Geometry check sheet. Reference: the model listing, model coordinates, mm. A direction names the side the tool comes from. Round coordinates to 2 decimals unless told otherwise and drop trailing zeros. Write each loop counter-clockwise with the first axis right and the second up, starting at its lowest first coordinate (ties: lowest second). Pieces come first, ordered by that corner, then holes. Notation, with made-up numbers: M -2,85 L 53,85 A29 cw 53,106 Z; hole C 26.5,-22.5 d8. An arc over 180 degrees is marked long. Use a Markdown table: item, result.
```python
from build123d import *

# Parameters (mm, degrees)
BOSS_EXTRUDE1_DEPTH = 34
SKETCH4_R           = 11
BOSS_EXTRUDE2_DEPTH = 1.5
SKETCH5_W           = 15
SKETCH5_H           = 6
BOSS_EXTRUDE3_DEPTH = 6
SKETCH6_R           = 9
CUT_EXTRUDE1_DEPTH  = 2
SKETCH7_R           = 2.5
BOSS_EXTRUDE4_DEPTH = 20
CUT_EXTRUDE3_DEPTH  = 20
FILLET1_R           = 1
FILLET2_R           = 1
SKETCH9_R           = 1.5
CUT_EXTRUDE4_DEPTH  = 20


with BuildPart() as part:
    # Sketch2 → Boss-Extrude1 (new body)
    with BuildSketch(Plane.XY):
        with BuildLine():
            Line((-16, -21), (16, -21))
            ThreePointArc((16, -21), (19.535533906, -19.535533906), (21, -16))
            Line((21, -16), (21, 16))
            ThreePointArc((21, 16), (19.535533906, 19.535533906), (16, 21))
            Line((16, 21), (-16, 21))
            ThreePointArc((-16, 21), (-19.535533906, 19.535533906), (-21, 16))
            Line((-21, 16), (-21, -16))
            ThreePointArc((-21, -16), (-19.535533906, -19.535533906), (-16, -21))
        make_face()
    extrude(amount=BOSS_EXTRUDE1_DEPTH)

    # Sketch4 → Boss-Extrude2 (add)
    with BuildSketch(Plane.XY.offset(34)):
        Circle(SKETCH4_R)
    extrude(amount=BOSS_EXTRUDE2_DEPTH)

    # Sketch5 → Boss-Extrude3 (add)
    with BuildSketch(Plane.XZ.offset(21)):
        with Locations((0, 7)):
            Rectangle(SKETCH5_W, SKETCH5_H)
    extrude(amount=BOSS_EXTRUDE3_DEPTH)

    # Sketch6 → Cut-Extrude1 (cut)
    with BuildSketch(Plane.XY.offset(35.5)):
        Circle(SKETCH6_R)
    extrude(amount=-CUT_EXTRUDE1_DEPTH, mode=Mode.SUBTRACT)

    # Sketch7 → Boss-Extrude4 (add)
    with BuildSketch(Plane.XY.offset(33.5)):
        Circle(SKETCH7_R)
    extrude(amount=BOSS_EXTRUDE4_DEPTH)

    # Sketch8 → Cut-Extrude3 (cut)
    with BuildSketch(Plane.XY.offset(27)):
        with BuildLine():
            Line((16, 21), (-16, 21))
            ThreePointArc((-16, 21), (-19.535533906, 19.535533906), (-21, 16))
            Line((-21, 16), (-21, -16))
            ThreePointArc((-21, -16), (-19.535533906, -19.535533906), (-16, -21))
            Line((-16, -21), (16, -21))
            ThreePointArc((16, -21), (19.535533906, -19.535533906), (21, -16))
            Line((21, -16), (21, 16))
            ThreePointArc((21, 16), (19.535533906, 19.535533906), (16, 21))
        make_face()
        with BuildLine():
            Line((16, 20.9), (-16, 20.9))
            ThreePointArc((-16, 20.9), (-19.464823228, 19.464823228), (-20.9, 16))
            Line((-20.9, 16), (-20.9, -16))
            ThreePointArc((-20.9, -16), (-19.464823228, -19.464823228), (-16, -20.9))
            Line((-16, -20.9), (16, -20.9))
            ThreePointArc((16, -20.9), (19.464823228, -19.464823228), (20.9, -16))
            Line((20.9, -16), (20.9, 16))
            ThreePointArc((20.9, 16), (19.464823228, 19.464823228), (16, 20.9))
        make_face(mode=Mode.SUBTRACT)
    extrude(amount=-CUT_EXTRUDE3_DEPTH, mode=Mode.SUBTRACT)

    # Fillet1
    fillet1_edges = [part.edges().sort_by_distance(p)[0] for p in [
        (-21, 0, 0),
        (-19.535533906, 19.535533906, 0),
        (0, 21, 0),
        (19.535533906, 19.535533906, 0),
        (-19.535533906, 19.535533906, 34),
        (-21, 0, 34),
        (-19.535533906, -19.535533906, 34),
        (0, -21, 34),
        (19.535533906, -19.535533906, 34),
        (21, 0, 34),
        (19.535533906, 19.535533906, 34),
        (21, 0, 0),
        (0, 21, 34),
        (19.535533906, -19.535533906, 0),
        (0, -21, 0),
        (-19.535533906, -19.535533906, 0),
    ]]
    fillet(fillet1_edges, radius=FILLET1_R)

    # Fillet2
    fillet2_edges = [part.edges().sort_by_distance(p)[0] for p in [
        (-2.5, 0, 53.5),
    ]]
    fillet(fillet2_edges, radius=FILLET2_R)

    # Sketch9 → Cut-Extrude4 (cut)
    with BuildSketch(Plane.XY.offset(34)):
        with Locations((15.5, 15.5)):
            Circle(SKETCH9_R)
        with Locations((15.5, -15.5)):
            Circle(SKETCH9_R)
        with Locations((-15.5, -15.5)):
            Circle(SKETCH9_R)
        with Locations((-15.5, 15.5)):
            Circle(SKETCH9_R)
    extrude(amount=-CUT_EXTRUDE4_DEPTH, mode=Mode.SUBTRACT)


solid = part.part
```
Item 1: Mould release check, pull along Y, two halves, no side actions. Record for faces 4 (the face through (20, 19, 4)), 5 (the face through (21, 0, 4)), 6 (the face through (19, -20, 30)), 7 (the face through (15, -15, 14)): +Y half, -Y half, draft (parallel to the pull), parting line (faces both ways), or undercut.
Outcome:
| item | result |
|---|---|
| face 4 | +Y half |
| face 5 | draft |
| face 6 | -Y half |
| face 7 | undercut |
Item 2: Access from +Z, -Z, +X, -X, +Y, -Y to the whole of each face (thin tool, end or side, straight path). Record for faces 1 (the face through (-19.5, -19.43, 17.14)), 2 (the face through (20.9, 0, 17)), 3 (the face through (7.5, -24, 7)).
Outcome:
| item | result |
|---|---|
| face 1 | -X, -Y |
| face 2 | +X, +Y, -Y |
| face 3 | +Z, -Z, +X, -Y |
Item 3: Material ranges on line 1 along Y through (x, z) = (0, 35); line 2 along Y through (x, z) = (15.5, 25.5); line 3 along X through (y, z) = (-15, 23), recorded low to high. Write a range as from..to.
Outcome:
| item | result |
|---|---|
| line 1 | y = -11..-9, -2.5..2.5, 9..11 |
| line 2 | y = -20.9..-17, -14..14, 17..20.9 |
| line 3 | x = -20.9..-16.91, -14.09..14.09, 16.91..20.9 |
Item 4: Go/stop test with flat-tipped pins: pin 1 (1.5 mm diameter, centred on y = -7.5, z = 21, fed in from -X); pin 2 (3 mm diameter, centred on x = 2, y = -24, fed in from +Z); pin 3 (1 mm diameter, centred on x = -15.5, z = 23.5, fed in from -Y). Record where each tip stops, or that it passes through.
Outcome:
| item | result |
|---|---|
| pin 1 | stops at x = -20.9 |
| pin 2 | stops at z = 10 |
| pin 3 | stops at y = -20.9 |
Item 5: Cross-section at A-A, the plane z = 15. Record the cut outline in (x, y), and give its area (3 significant figures).
Outcome:
| item | result |
|---|---|
| outline | M -20.9,-16 A4.9 ccw -16,-20.9 L 16,-20.9 A4.9 ccw 20.9,-16 L 20.9,16 A4.9 ccw 16,20.9 L -16,20.9 A4.9 ccw -20.9,16 Z; hole C -15.5,-15.5 d3; hole C -15.5,15.5 d3; hole C 15.5,-15.5 d3; hole C 15.5,15.5 d3 |
| area | 1,700 mm2 |
Item 6: Cross-section at D-D, the plane y = -12. Record the cut outline in (x, z), and give its area (3 significant figures).
Outcome:
| item | result |
|---|---|
| outline | M -21,1 A1 ccw -20,0 L 20,0 A1 ccw 21,1 L 21,7 L 20.9,7 L 20.9,27 L 21,27 L 21,33 A1 ccw 20,34 L -20,34 A1 ccw -21,33 L -21,27 L -20.9,27 L -20.9,7 L -21,7 Z |
| area | 1,420 mm2 |
